Drawing for the job (mm, zero at the part's lowest x, y, z). Give positions to 0.01 mm unless a question says otherwise; leave off trailing zeros. Write each loop counter-clockwise with the first axis right and the second up, starting at its lowest first coordinate (ties: lowest second). Pieces come first, ordered by that corner, then holes. Notation, with made-up numbers: (-14, 34.5) - (9, 34.5) arc R25 cw to (9, 49.5) - close; hole circle Ø1 at (20.5, 58.25). An arc over 180 degrees is marked (long way). Write item = value, one per line. Start each with the question number.
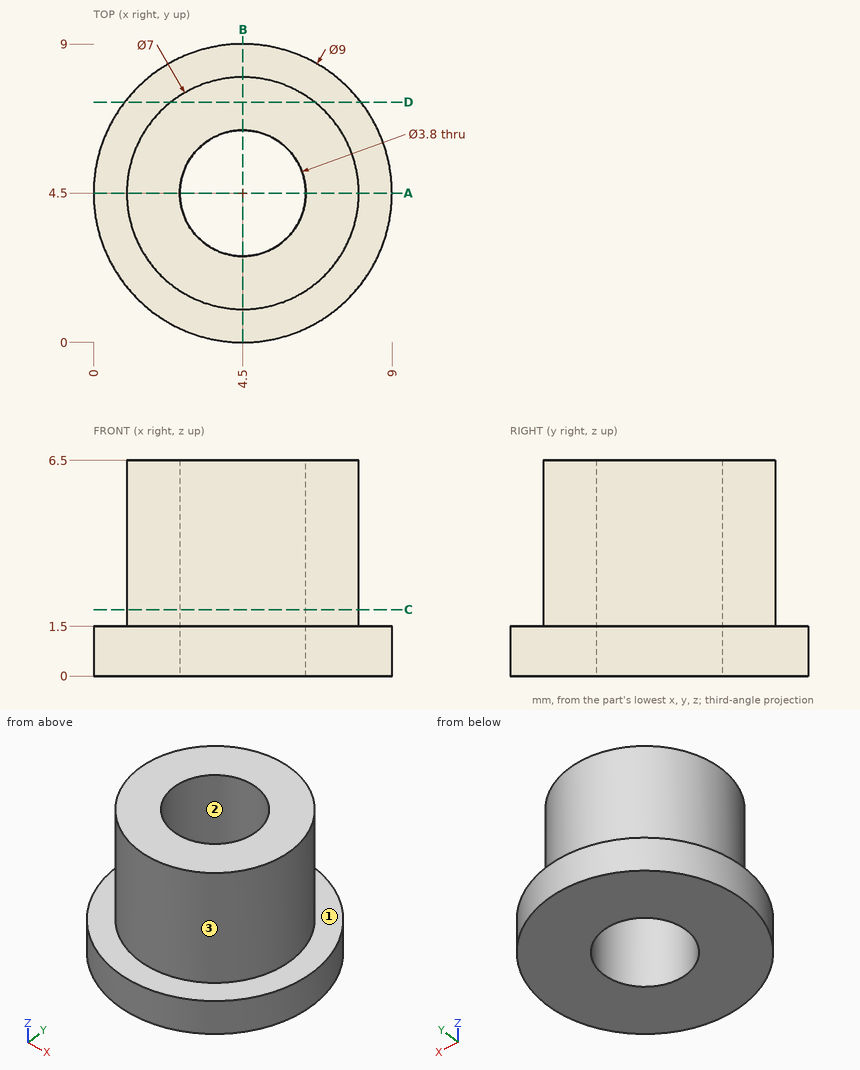
1. Cut at D-D (y = 7.25). Give the cut face in (x, z), then the cut area to 3 significant figures.
2. Mould opens along X. For the marked faces 1, 2 and 3 say: +X half, -X half, draft (parallel to the pull), parting line (faces both ways), or undercut.
3. Wall check: line 1 along Y through (x, z) = (4.5, 3.75); line 2 along Z through (x, y) = (6.5, 7.5); line 3 along Y through (x, z) = (5.75, 2). Give the ranges that are in metal, low to high.
4. Cut at A-A (y = 4.5). Give the cut face in (x, z).
5. Cut at C-C (z = 2). Give the cut face in (x, y).
6. Pin check, flat tips, straight feed: pin 1 Ø1.5 at (x, z) = (7.5, 5) entering from -Y; pin 2 Ø2 at (y, z) = (2, 5.5) entering from -X; pin 3 Ø1.5 at (y, z) = (4.5, 2.5) entering from +X; pin 4 Ø3.5 at (x, y) = (4.5, 4.5) entering from -Z. Stop position of each tip, or through.
Output:
q1.outline = (0.94, 0) - (8.06, 0) - (8.06, 1.5) - (6.67, 1.5) - (6.67, 6.5) - (2.33, 6.5) - (2.33, 1.5) - (0.94, 1.5) - close
q1.area = 32.3 mm2
q2.face_1 = draft
q2.face_2 = undercut
q2.face_3 = parting line
q3.line_1 = 1 to 2.6, 6.4 to 8
q3.line_2 = 0 to 1.5
q3.line_3 = 1.23 to 3.07, 5.93 to 7.77
q4.outline = (0, 0) - (2.6, 0) - (2.6, 6.5) - (1, 6.5) - (1, 1.5) - (0, 1.5) - close; (6.4, 0) - (9, 0) - (9, 1.5) - (8, 1.5) - (8, 6.5) - (6.4, 6.5) - close
q5.outline = circle Ø7 at (4.5, 4.5); hole circle Ø3.8 at (4.5, 4.5)
q6.pin_1 = 1.82
q6.pin_2 = 1.34
q6.pin_3 = 8
q6.pin_4 = through
